The model under review builds one solid part; all positions refer to its coordinate system, in mm. A direction names the side the tool comes from. Round coordinates to 2 decimals unless told otherwise and drop trailing zeros. Loops run counter-clockwise (first coordinate to the right, second up) from the corner with the lowest first, then second, coordinate; pieces in that order, holes last. Notation, with made-up numbers: (12.25, 71) - (50.25, 71) arc R7 ccw to (50.25, 76) - close; hole circle Ø4 at (86, 85.25). An arc over 180 degrees is marked (long way). Answer as CSV lines item,"result".
Autodesk Inventor part; units mm, degrees
ref_plane "YZ Plane" through (0, 0, 0) normal (1, 0, 0) x (0, 1, 0)
ref_plane "XZ Plane" through (0, 0, 0) normal (0, 1, 0) x (-1, 0, 0)
ref_plane "XY Plane" through (0, 0, 0) normal (0, 0, 1) x (1, 0, 0)
sketch "Sketch1" plane through (0, 0, 0) normal (1, 0, 0) x (0, 1, 0)
  line L0 (0, 0) -> (0, -41.9923)
  line L1 (35.5, 0) -> (22.4345, 0)
  line L2 (22.4345, 0) -> (22.4345, -9.2803)
  line L3 (22.4345, -9.2803) -> (35.5, -9.2803)
  arc A0 (35.5, -9.2803) -> (35.5, 0) centre (27.6519, -4.6401) ccw
revolve "Revolution1" add sketch "Sketch1" angle 330 about axis through (0, 0, 0) along (0, 0, -1)
sketch "Sketch2" plane through (0, 22.4345, 0) normal (0, 0, 1) x (1, 0, 0)
  arc A0 (-11.2172, -3.0056) -> (0, 0) centre (0, -22.4345) ccw
  arc A1 (-15.1658, 3.8334) -> (0, 7.8971) centre (0, -22.4345) ccw
  line L0 (-11.2172, -3.0056) -> (-15.1658, 3.8334)
  line L1 (-17.75, 8.3094) -> (-11.2172, -3.0056)
  line L2 (0, 7.8971) -> (0, 0)
  point P0 (0, -22.4345)
extrude "Extrusion1" add sketch "Sketch2" along normal blind 11.5
properties part number "SPRING SUPPORT"
1. Wall thickness on probe 1 along X at (y, z) = (-4, 9) (3 decimals); probe 2 along Y at (x, z) = (1.5, -5.25); probe 3 along Y at (x, z) = (-18, 10.5): over which ranges is each line inside the solid? List them lowest first.
Numbers:
probe 1,"x = -30.067 to -22.075, 22.075 to 30.067"
probe 2,"y = -36.72 to -22.38, 22.38 to 36.72"
probe 3,"y = -24.41 to -13.39, 13.39 to 24.41"
2. Take a section at A-A (y = 0). State the section outline as (x, z) points.
Numbers:
outline,"(-35.5, -9.28) - (-22.43, -9.28) - (-22.43, 11.5) - (-30.33, 11.5) - (-30.33, 0) - (-35.5, 0) arc R9.12 ccw to start; (22.43, -9.28) - (35.5, -9.28) arc R9.12 ccw to (35.5, 0) - (30.33, 0) - (30.33, 11.5) - (22.43, 11.5) - close"
3. Take a section at C-C (z = 9.75). State the section outline as (x, y) points, plus the area to 3 significant figures.
Numbers:
outline,"(-15.17, 26.27) arc R30.33 ccw (long way) to (0, 30.33) - (0, 22.43) arc R22.43 cw (long way) to (-11.22, 19.43) - close"
area,"1,200 mm²"
4. Tool access review of faces 1 (the face through (6.675, -21.418, 5.67)), 2 (the face through (11, -29, 0)): name each direction out of +Z, -Z, +X, -X, +Y, -Y from which nothing blocks a thin tool from reaching the whole face with its end or side.
Numbers:
face 1,"+Z, -Z"
face 2,"+Z"
5. Clearance check with flat-ended pins moving along their axes: pin 1 (2 mm diameter, centred on x = -24, y = -20.5, fed in from +Z); pin 2 (6 mm diameter, centred on x = -25, y = 19, fed in from +Z); pin 3 (1.5 mm diameter, centred on y = 22.5, z = 8, fed in from +X); pin 4 (1.5 mm diameter, centred on y = -1, z = 2, fed in from +X). State where each tip first meets the part, or that it passes through.
Numbers:
pin 1,"stops at z = 0"
pin 2,"stops at z = 11.5"
pin 3,"stops at x = 21.14"
pin 4,"stops at x = 30.33"
6. Draft analysis for pull direction X (two halves, no side actions). For faces 3 (the face through (0, 28, -1)), 4 (the face through (-4.6, -22.3, 11.5)), 5 (the face through (6.675, -21.418, -4.705)), 6 (the face through (9.025, -28.958, 5.67)), state which applies: +X half, -X half, draft (parallel to the pull), parting line (faces both ways), or undercut.
Numbers:
face 3,"undercut"
face 4,"draft"
face 5,"undercut"
face 6,"parting line"
7. Take a section at B-B (z = -3.75). State the section outline as (x, y) points, plus the area to 3 significant figures.
Numbers:
outline,"(-18.36, 31.81) arc R36.73 ccw (long way) to (0, 36.73) - (0, 22.43) arc R22.43 cw (long way) to (-11.22, 19.43) - close"
area,"2,430 mm²"
